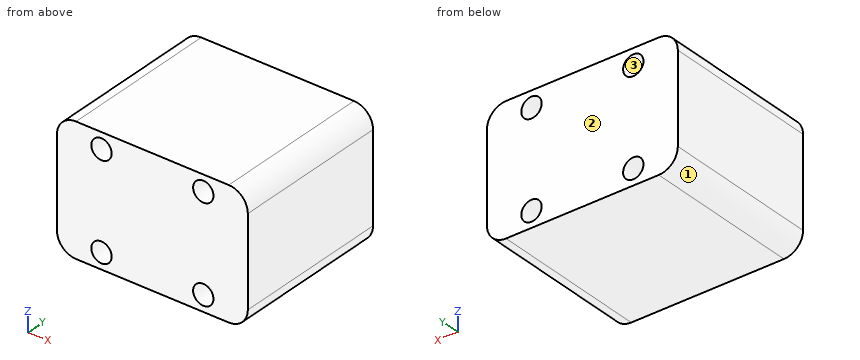
```python
from build123d import *

# Parameters (mm, degrees)
SKETCH_1_W      = 30
SKETCH_1_H      = 20
SKETCH_1_R      = 1.6
EXTRUDE_1_DEPTH = 25
FILLET_1_R      = 3


with BuildPart() as part:
    # 草图1 → 凸台-拉伸1 (new body)
    with BuildSketch(Plane(origin=(0, 0, 0), x_dir=(1, 0, 0), z_dir=(0, 1, 0))):
        Rectangle(SKETCH_1_W, SKETCH_1_H)
        with Locations((-8, 7.5)):
            Circle(SKETCH_1_R, mode=Mode.SUBTRACT)
        with Locations((-8, -7.5)):
            Circle(SKETCH_1_R, mode=Mode.SUBTRACT)
        with Locations((8, -7.5)):
            Circle(SKETCH_1_R, mode=Mode.SUBTRACT)
        with Locations((8, 7.5)):
            Circle(SKETCH_1_R, mode=Mode.SUBTRACT)
    extrude(amount=EXTRUDE_1_DEPTH)

    # 圆角1
    fillet_1_edges = [part.edges().sort_by_distance(p)[0] for p in [
        (15, 12.5, 10),
        (-15, 12.5, 10),
        (-15, 12.5, -10),
        (15, 12.5, -10),
    ]]
    fillet(fillet_1_edges, radius=FILLET_1_R)


solid = part.part
```
CAD build for the part. Positions are in the model's coordinates, mm. Face numbers are marked on the shaded views. Coordinates: 2 decimals unless noted, no trailing zeros. Write each loop counter-clockwise with the first axis right and the second up, starting at its lowest first coordinate (ties: lowest second). Pieces come first, ordered by that corner, then holes. Notation, with made-up numbers: (44, -40) -> (78, -40) arc R9 cw to (78, -31) -> close; hole circle Ø7 at (14.5, -12.75). An arc over 180 degrees is marked (long way). Use CSV: the item, a comma, the result in double quotes. Start each with the question number.
Item 1: Band-saw the part on C-C, the plane z = 7.5. Write the cut outline in (x, y).
Item 2: Wall check: probe 1 along Z at (x, y) = (8, 15.25); probe 2 along Z at (x, y) = (7.25, 11); probe 3 along X at (y, z) = (13.5, 7.5). Give the ranges that are in metal, low to high.
Item 3: Band-saw the part on B-B, the plane x = -8. Write the cut outline in (y, z), plus the area to 3 significant figures.
Item 4: Band-saw the part on A-A, the plane y = 10. Write the cut outline in (x, z), plus the area to 3 significant figures.
Item 5: Drop a flat-ended pin along its axis: P1, Ø4, axis at x = 8, z = -7.5, coming from the +Y side. Give the stop position or say it passes through.
Item 6: Two-plate mould, pull along X, no slides. Class the marked faces 1, 2 and 3: +X half, -X half, draft (parallel to the pull), parting line (faces both ways), or undercut.
Response values:
1,outline,"(-14.96, 0) -> (-9.6, 0) -> (-9.6, 25) -> (-14.96, 25) -> close; (-6.4, 0) -> (6.4, 0) -> (6.4, 25) -> (-6.4, 25) -> close; (9.6, 0) -> (14.96, 0) -> (14.96, 25) -> (9.6, 25) -> close"
2,probe 1,"z = -10 to -9.1, -5.9 to 5.9, 9.1 to 10"
2,probe 2,"z = -10 to -8.91, -6.09 to 6.09, 8.91 to 10"
2,probe 3,"x = -14.96 to -9.6, -6.4 to 6.4, 9.6 to 14.96"
3,outline,"(0, -10) -> (25, -10) -> (25, -9.1) -> (0, -9.1) -> close; (0, -5.9) -> (25, -5.9) -> (25, 5.9) -> (0, 5.9) -> close; (0, 9.1) -> (25, 9.1) -> (25, 10) -> (0, 10) -> close"
3,area,"340 mm2"
4,outline,"(-15, -7) arc R3 ccw to (-12, -10) -> (12, -10) arc R3 ccw to (15, -7) -> (15, 7) arc R3 ccw to (12, 10) -> (-12, 10) arc R3 ccw to (-15, 7) -> close; hole circle Ø3.2 at (-8, -7.5); hole circle Ø3.2 at (-8, 7.5); hole circle Ø3.2 at (8, -7.5); hole circle Ø3.2 at (8, 7.5)"
4,area,"560 mm2"
5,P1,"stops at y = 25"
6,face 1,"-X half"
6,face 2,"draft"
6,face 3,"undercut"
